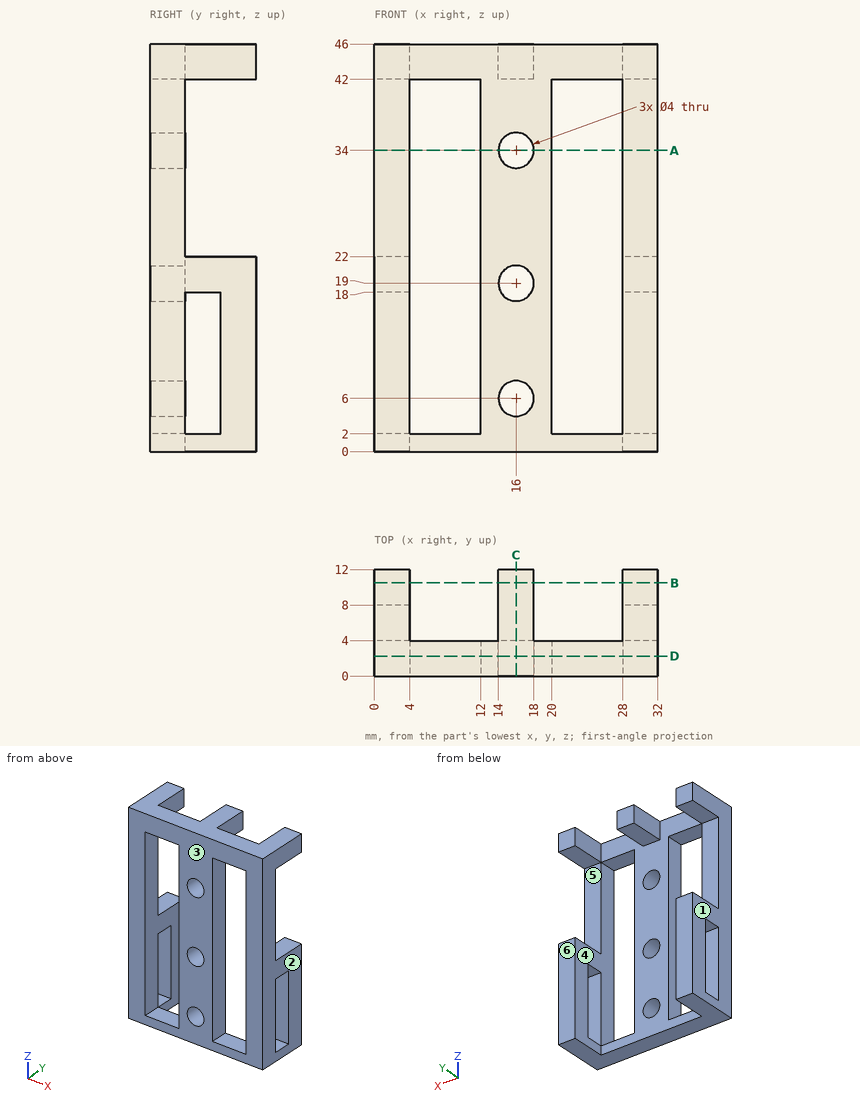
Drawing for the job (mm, zero at the part's lowest x, y, z). A direction names the side the tool comes from. Round coordinates to 2 decimals unless told otherwise and drop trailing zeros. Write each loop counter-clockwise with the first axis right and the second up, starting at its lowest first coordinate (ties: lowest second). Pieces come first, ordered by that corner, then holes. Notation, with made-up numbers: (80.25, -20) - (118.25, -20) arc R23 ccw to (118.25, 12) - close; hole circle Ø3 at (-2, 55.25). An arc over 180 degrees is marked (long way). Write item = value, one per line. Start each with the question number.
Q1. Band-saw the part on A-A (z = 34). Give the cut face in (x, y).
Q2. Probe L1, parallel to Z at x = 16, y = 3.05; L2, parallel to X at y = 3, z = 3.5; L3, parallel to X at y = 10.25, z = 19. List the from-to ranges inside material, lowest first. Write a range as from..to.
Q3. Band-saw the part on D-D (y = 2.25). Give the cut face in (x, z), then the cut area to 3 significant figures.
Q4. Drop flat-ended pins along their axis: pin 1 (6.5 mm diameter, centred on x = 16, z = 19, fed in from +Y); pin 2 (2 mm diameter, centred on x = 16, y = 8.5, fed in from -Z). Give the stop position or say it passes through.
Q5. Band-saw the part on B-B (y = 10.5). Give the cut face in (x, z), then the cut area to 3 significant figures.
Q6. Mould opens along X. For the marked faces 1, 2, 3 and 4 say: pulls with the +X half, pulls with the -X half, needs draft (parallel to the pull), parting line crosses it, or undercut.
Q7. Which spindle directions (+Z, -Z, +X, -X, +Y, -Y) get a long thin tool onto all of the face, cutting with end or side? Do the marked faces 5 and 6. Say none if no direction does.
Q8. Band-saw the part on C-C (x = 16). Give the cut face in (y, z), then the cut area to 3 significant figures.
Answers below:
q1.outline = (0, 0) - (4, 0) - (4, 4) - (0, 4) - close; (12, 0) - (14, 0) - (14, 4) - (12, 4) - close; (18, 0) - (20, 0) - (20, 4) - (18, 4) - close; (28, 0) - (32, 0) - (32, 4) - (28, 4) - close
q2.L1 = 0..4, 8..17, 21..32, 36..46
q2.L2 = 0..4, 12..20, 28..32
q2.L3 = 0..4, 28..32
q3.outline = (0, 0) - (32, 0) - (32, 46) - (0, 46) - close; hole (4, 2) - (12, 2) - (12, 42) - (4, 42) - close; hole circle Ø4 at (16, 6); hole circle Ø4 at (16, 19); hole circle Ø4 at (16, 34); hole (20, 2) - (28, 2) - (28, 42) - (20, 42) - close
q3.area = 794 mm2
q4.pin_1 = 4
q4.pin_2 = 42
q5.outline = (0, 0) - (4, 0) - (4, 22) - (0, 22) - close; (0, 42) - (4, 42) - (4, 46) - (0, 46) - close; (14, 42) - (18, 42) - (18, 46) - (14, 46) - close; (28, 0) - (32, 0) - (32, 22) - (28, 22) - close; (28, 42) - (32, 42) - (32, 46) - (28, 46) - close
q5.area = 224 mm2
q6.face_1 = pulls with the -X half
q6.face_2 = pulls with the +X half
q6.face_3 = needs draft
q6.face_4 = undercut
q7.face_5 = +X, -X, +Y
q7.face_6 = +Z, -Z, +X, -X, +Y
q8.outline = (0, 0) - (4, 0) - (4, 4) - (0, 4) - close; (0, 8) - (4, 8) - (4, 17) - (0, 17) - close; (0, 21) - (4, 21) - (4, 32) - (0, 32) - close; (0, 36) - (4, 36) - (4, 42) - (12, 42) - (12, 46) - (0, 46) - close
q8.area = 168 mm2
